CAD build for the part. Positions are in the model's coordinates, mm. A direction names the side the tool comes from. Coordinates: 2 decimals unless noted, no trailing zeros. Loops run counter-clockwise (first coordinate to the right, second up) from the corner with the lowest first, then second, coordinate; pieces in that order, holes last. Notation, with made-up numbers: (48.5, -4) -> (54.5, -4) arc R18 cw to (54.5, 27) -> close; hole circle Ø5 at (34, -36). An arc over 180 degrees is marked (long way). Answer as a JSON object with one key per item and string values. Group by question number.
from build123d import *

# Parameters (mm, degrees)
F0_W     = 152.4
F0_H     = 152.4
F0_R     = 38.1
F1_DEPTH = 101.6
F2_R     = 57.15
F2_R_2   = 38.1
F3_DEPTH = 9.525
F4_R     = 57.15
F4_R_2   = 38.1
F5_DEPTH = 9.525


with BuildPart() as f1:
    # F0 (on Front) → F1 (new body)
    with BuildSketch(Plane.XZ):
        Rectangle(F0_W, F0_H)
        Circle(F0_R, mode=Mode.SUBTRACT)
    extrude(amount=F1_DEPTH)

    # F2 (on face) → F3 (join)
    with BuildSketch(Plane.XZ.offset(101.6)):
        Circle(F2_R)
        Circle(F2_R_2, mode=Mode.SUBTRACT)
    extrude(amount=F3_DEPTH)

    # F4 (on face) → F5 (join)
    with BuildSketch(Plane(origin=(0, 0, 0), x_dir=(-1, 0, 0), z_dir=(0, 1, 0))):
        Circle(F4_R)
        Circle(F4_R_2, mode=Mode.SUBTRACT)
    extrude(amount=F5_DEPTH)


solid = f1.part
Item 1: Band-saw the part on D-D, the plane z = -55. List the corners of the cut face in (x, y) (3 decimals), and give its area (3 significant figures).
Item 2: Band-saw the part on B-B, the plane x = 0. List the corners of the cut face in (y, z) (3 decimals), and give its area (3 significant figures).
Item 3: Band-saw the part on C-C, the plane z = 0. List the corners of the cut face in (x, y) (3 decimals).
Item 4: Flat gauge pin, fed straight in: P1, Ø5, axis at x = 20, z = -59.5, coming from the +Y side. Where does the tip first touch, or does it go through?
Item 5: Drill centre lines: L1, parallel to X at y = -81, z = 0; L2, parallel to Z at x = 0, y = 6. Where is each one in solid material? Low to high.
Item 6: Band-saw the part on A-A, the plane y = -88. List the corners of the cut face in (x, z).
Item 7: 3-axis set-ups, long thin cutter, end or side, ignore diameter. For faces 1 (the flat face through (33, 0, 52)), 2 (the flat face through (33, -101.6, 52)), 3 (the flat face through (76.2, -50, -1)): which of +Z, -Z, +X, -X, +Y, -Y reach the whole face in a straight line?
Reply:
{
 "1": {"outline": "(-76.2, -101.6) -> (-15.528, -101.6) -> (-15.528, -111.125) -> (15.528, -111.125) -> (15.528, -101.6) -> (76.2, -101.6) -> (76.2, 0) -> (15.528, 0) -> (15.528, 9.525) -> (-15.528, 9.525) -> (-15.528, 0) -> (-76.2, 0) -> close", "area": "16,100 mm²"},
 "2": {"outline": "(-111.125, -57.15) -> (-101.6, -57.15) -> (-101.6, -76.2) -> (0, -76.2) -> (0, -57.15) -> (9.525, -57.15) -> (9.525, -38.1) -> (-111.125, -38.1) -> close; (-111.125, 38.1) -> (9.525, 38.1) -> (9.525, 57.15) -> (0, 57.15) -> (0, 76.2) -> (-101.6, 76.2) -> (-101.6, 57.15) -> (-111.125, 57.15) -> close", "area": "8,470 mm²"},
 "3": {"outline": "(-76.2, -101.6) -> (-57.15, -101.6) -> (-57.15, -111.125) -> (-38.1, -111.125) -> (-38.1, 9.525) -> (-57.15, 9.525) -> (-57.15, 0) -> (-76.2, 0) -> close; (38.1, -111.125) -> (57.15, -111.125) -> (57.15, -101.6) -> (76.2, -101.6) -> (76.2, 0) -> (57.15, 0) -> (57.15, 9.525) -> (38.1, 9.525) -> close"},
 "4": {"P1": "y = 0"},
 "5": {"L1": "-76.2 to -38.1, 38.1 to 76.2", "L2": "-57.15 to -38.1, 38.1 to 57.15"},
 "6": {"outline": "(-76.2, -76.2) -> (76.2, -76.2) -> (76.2, 76.2) -> (-76.2, 76.2) -> close; hole circle Ø76.2 at (0, 0)"},
 "7": {"face 1": "+Y", "face 2": "-Y", "face 3": "+Z, -Z, +X, +Y, -Y"}
}
